For this review, take the finished solid that the model builds, in its own axes (mm). Face numbers are marked on the shaded views. A direction names the side the tool comes from. Round coordinates to 2 decimals unless told otherwise and drop trailing zeros. Order: outer loops, then holes, each group sorted by start corner. A loop starts at its lowest first (then second) coordinate and runs counter-clockwise, first axis right, second up. Notation, with made-up numbers: (-7, -23) -> (15, -23) arc R20 cw to (15, -18) -> close; hole circle Ø11 at (0.25, 87.25). An arc over 180 degrees is marked (long way). Use a Markdown table: item, result. Add a question column.
1) Wall thickness on line 1 along Z through (x, y) = (-115, 7.5); line 2 along X through (y, z) = (20.5, 12); line 3 along X through (y, z) = (24, 16): over which ranges is each line inside the solid? List them lowest first. Write a range as [from, to].
2) Clearance check with flat-ended pins moving along their axes: P1, Ø4, axis at x = -282, y = 7.5, coming from the -Z side; P2, Ø6, axis at y = 7, z = 52, coming from the -X side; P3, Ø4, axis at y = 7.5, z = 73.5, coming from the +X side. State where each tip first meets the part, or that it passes through.
3) Consider section B-B (y = 5.25). State the section outline as (x, z) points, plus the area to 3 significant figures.
4) Machinability: for the marked faces 1 and 2, which of the approach directions +Z, -Z, +X, -X, +Y, -Y give a long, thin tool a straight path to every point of the face, cutting with its end or side? Answer none if there is none.
5) Draft analysis for pull direction X (two halves, no side actions). For the marked faces 3, 4, 5 and 6, state which applies: pulls with the +X half, pulls with the -X half, needs draft (parallel to the pull), parting line crosses it, or undercut.
6) Consider section A-A (z = 87). State the section outline as (x, y) points, plus the area to 3 significant figures.
7) Consider section C-C (z = 71.5). State the section outline as (x, y) points.
8) Consider section D-D (x = -313). State the section outline as (y, z) points, plus the area to 3 significant figures.
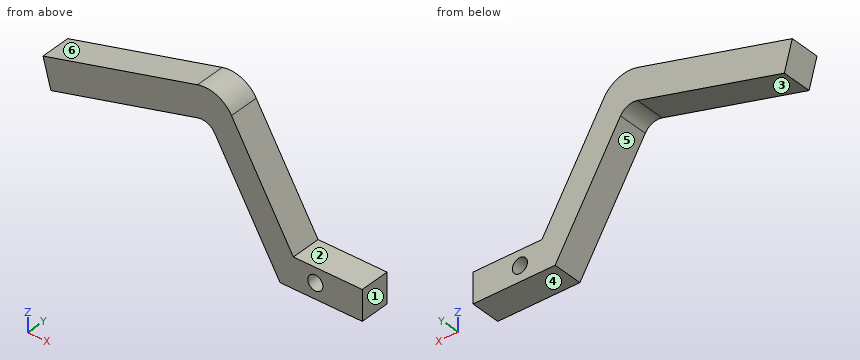
Autodesk Inventor part; units mm, degrees
ref_plane "YZ Plane" through (0, 0, 0) normal (1, 0, 0) x (0, 1, 0)
ref_plane "XZ Plane" through (0, 0, 0) normal (0, 1, 0) x (-1, 0, 0)
ref_plane "XY Plane" through (0, 0, 0) normal (0, 0, 1) x (1, 0, 0)
sketch "Sketch2" plane through (0, 0, 0) normal (0, 1, 0) x (-1, 0, 0)
  line L0 (69.0728, 25.4) -> (127, 25.4)
  line L1 (127, 25.4) -> (179.0216, 114.7196)
  line L2 (207.6006, 126.4556) -> (337.4623, 91.34)
  line L3 (337.4623, 91.34) -> (330.8321, 66.8206)
  line L4 (330.8321, 66.8206) -> (207.3781, 100.2035)
  line L5 (193.0887, 94.3355) -> (138.1457, 0)
  line L6 (138.1457, 0) -> (69.0728, 0)
  arc A0 (207.3781, 100.2035) -> (193.0887, 94.3355) centre (204.063, 87.9438) ccw
  arc A1 (207.6006, 126.4556) -> (179.0216, 114.7196) centre (200.9703, 101.9363) ccw
  line L7 (69.0728, 25.4) -> (69.0728, 0)
  point P0 (0, 0)
  dimension "d6" = 25.4
  dimension "d7" = 12.7
  dimension "d8" = 25.4
extrude "Extrusion1" add sketch "Sketch2" along normal blind 25.4
sketch "Sketch3" plane through (0, 25.4, 0) normal (0, 1, 0) x (1, 0, 0)
  point P0 (0, 0)
  point P1 (-108.5039, -12.9749)
hole "Hole1" at (-108.5039, 25.4, 12.9749) direction (0, -1, 0) diameter 12.7 depth 38.1 tip angle 118
properties part number "Scissor"
Results list:
| question | item | result |
|---|---|---|
| 1 | line 1 | [0, 25.4] |
| 1 | line 2 | [-145.13, -114.78], [-102.23, -69.07] |
| 1 | line 3 | [-147.46, -114.09], [-102.92, -69.07] |
| 2 | P1 | z = 79.48 |
| 2 | P2 | x = -170.18 |
| 2 | P3 | x = -153.85 |
| 3 | outline | (-337.46, 91.34) -> (-330.83, 66.82) -> (-207.38, 100.2) arc R12.7 cw to (-193.09, 94.34) -> (-138.15, 0) -> (-69.07, 0) -> (-69.07, 25.4) -> (-127, 25.4) -> (-179.02, 114.72) arc R25.4 ccw to (-207.6, 126.46) -> close; hole circle Ø12.7 at (-108.5, 12.97) |
| 3 | area | 7,840 mm2 |
| 4 | face 1 | +Z, -Z, +X, +Y, -Y |
| 4 | face 2 | +Z, +X, +Y, -Y |
| 5 | face 3 | undercut |
| 5 | face 4 | needs draft |
| 5 | face 5 | undercut |
| 5 | face 6 | pulls with the -X half |
| 6 | outline | (-336.29, 0) -> (-256.21, 0) -> (-256.21, 25.4) -> (-336.29, 25.4) -> close; (-188.82, 0) -> (-162.88, 0) -> (-162.88, 25.4) -> (-188.82, 25.4) -> close |
| 6 | area | 2,690 mm2 |
| 7 | outline | (-332.1, 0) -> (-313.53, 0) -> (-313.53, 25.4) -> (-332.1, 25.4) -> close; (-179.79, 0) -> (-153.85, 0) -> (-153.85, 25.4) -> (-179.79, 25.4) -> close |
| 8 | outline | (0, 71.64) -> (25.4, 71.64) -> (25.4, 97.95) -> (0, 97.95) -> close |
| 8 | area | 668 mm2 |
